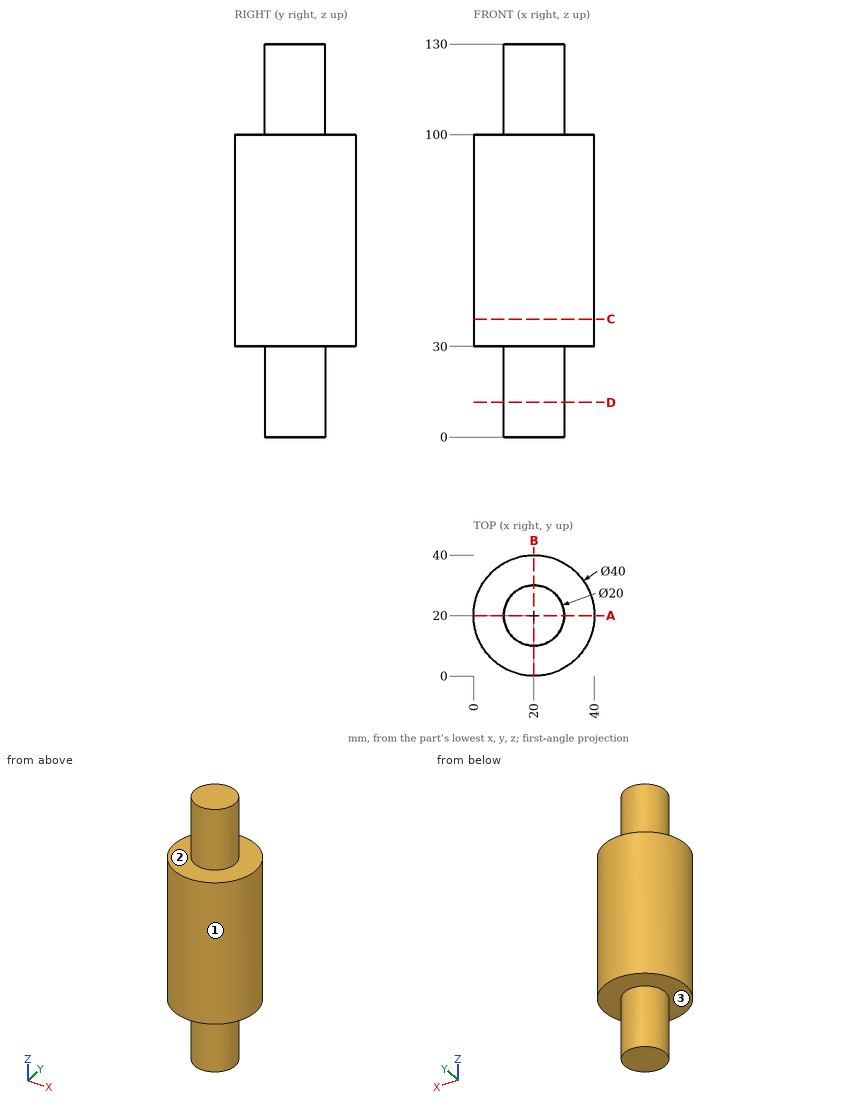
Can you work these out from the drawing? Everything is in mm from the part's minimum corner. A direction names the side the tool comes from. Round coordinates to 2 decimals unless told otherwise and drop trailing zeros. Loops run counter-clockwise (first coordinate to the right, second up) from the corner with the lowest first, then second, coordinate; pieces in that order, holes last. Notation, with made-up numbers: (2, -21.75) -> (10, -21.75) arc R15 cw to (10, -17.75) -> close; hole circle Ø11 at (2, 64.5). An arc over 180 degrees is marked (long way). Use CSV: the item, a comma, the result in double quotes.
(1) If I drill on probe 1 along Z at (x, y) = (37.5, 12.5); probe 2 along X at (y, z) = (16, 91.5); probe 3 along X at (y, z) = (22, 48.5), over which ranges is the centre line in solid material (lowest first)? Write a range as [from, to].
Return value:
probe 1,"z = [30, 100]"
probe 2,"x = [0.4, 39.6]"
probe 3,"x = [0.1, 39.9]"
(2) For the marked faces 1, 2 and 3, which set-ups out of +Z, -Z, +X, -X, +Y, -Y let a thin tool reach every point of the face, with its end or its side?
Return value:
face 1,"+Z, -Z"
face 2,"+Z"
face 3,"-Z"
(3) Suppose I cut it at A-A on y = 20. Write out the boundary of the cut face in (x, z), plus the area to 3 significant figures.
Return value:
outline,"(0, 30) -> (10, 30) -> (10, 0) -> (30, 0) -> (30, 30) -> (40, 30) -> (40, 100) -> (30, 100) -> (30, 130) -> (10, 130) -> (10, 100) -> (0, 100) -> close"
area,"4,000 mm²"
(4) Suppose I cut it at D-D on z = 11.5. Write out the boundary of the cut face in (x, y).
Return value:
outline,"circle Ø20 at (20, 20)"
(5) Will these pins go through, and if not, where does the flat tip stop? pin 1 Ø6 at (y, z) = (24.5, 49.5) entering from -X; pin 2 Ø1 at (y, z) = (13, 64) entering from +X; pin 3 Ø1.5 at (x, y) = (33.5, 6.5) entering from +Z.
Return value:
pin 1,"stops at x = 0.06"
pin 2,"stops at x = 38.91"
pin 3,"stops at z = 100"
(6) Suppose I cut it at C-C on z = 39. Write out the boundary of the cut face in (x, y), plus the area to 3 significant figures.
Return value:
outline,"circle Ø40 at (20, 20)"
area,"1,260 mm²"
